CAD build for the part. Positions are in the model's coordinates, mm. A direction names the side the tool comes from. Round coordinates to 2 decimals unless told otherwise and drop trailing zeros. Order: outer loops, then holes, each group sorted by start corner. A loop starts at its lowest first (then second) coordinate and runs counter-clockwise, first axis right, second up. Notation, with made-up numbers: (44, -30.75) - (59, -30.75) arc R24 cw to (59, 4.25) - close; hole circle Ø2 at (32.25, 16.25). An arc over 180 degrees is marked (long way). Write item = value, one per line.
from build123d import *

# Parameters (mm, degrees)
SKETCH1_W           = 155
SKETCH1_H           = 32
BOSS_EXTRUDE1_DEPTH = 2
SKETCH2_W           = 155
SKETCH2_H           = 2
SKETCH2_W_2         = 130
BOSS_EXTRUDE2_DEPTH = 6.25
CUT_EXTRUDE1_DEPTH  = 6.25
SKETCH4_R           = 1.5
CUT_EXTRUDE2_DEPTH  = 6.25
SKETCH5_R           = 2.875
CUT_EXTRUDE3_DEPTH  = 6.25
SKETCH6_R           = 1.5
CUT_EXTRUDE4_DEPTH  = 6
CHAMFER1_SIZE       = 1.5


with BuildPart() as part:
    # Sketch1 → Boss-Extrude1 (new body)
    with BuildSketch(Plane.XY):
        with Locations((77.5, -16)):
            Rectangle(SKETCH1_W, SKETCH1_H)
    extrude(amount=BOSS_EXTRUDE1_DEPTH)

    # Sketch2 → Boss-Extrude2 (add)
    with BuildSketch(Plane.XY.offset(2)):
        with Locations((77.5, -1)):
            Rectangle(SKETCH2_W, SKETCH2_H)
        with Locations((90, -23)):
            Rectangle(SKETCH2_W_2, SKETCH2_H)
    extrude(amount=BOSS_EXTRUDE2_DEPTH)

    # Sketch3 → Cut-Extrude1 (cut)
    with BuildSketch(Plane.XY.offset(2)):
        Polygon((155, -32), (23, -32), (23, -24), (23, -20.25), (25, -20.25), (25, -24), (155, -24), align=None)
    extrude(amount=-CUT_EXTRUDE1_DEPTH, mode=Mode.SUBTRACT)

    # Sketch4 → Cut-Extrude2 (cut)
    with BuildSketch(Plane.XY.offset(2)):
        with Locations((4.75, -27.5)):
            Circle(SKETCH4_R)
        with Locations((4.75, -17.5)):
            Circle(SKETCH4_R)
        with Locations((4.75, -7.5)):
            Circle(SKETCH4_R)
    extrude(amount=-CUT_EXTRUDE2_DEPTH, mode=Mode.SUBTRACT)

    # Sketch5 → Cut-Extrude3 (cut)
    with BuildSketch(Plane.XY.offset(2)):
        with Locations((130.075, -12)):
            Circle(SKETCH5_R)
        with Locations((100.025, -12)):
            Circle(SKETCH5_R)
        with Locations((80.025, -12)):
            Circle(SKETCH5_R)
        with Locations((49.925, -12)):
            Circle(SKETCH5_R)
    extrude(amount=-CUT_EXTRUDE3_DEPTH, mode=Mode.SUBTRACT)

    # Sketch6 → Cut-Extrude4 (cut)
    with BuildSketch(Plane.XY.offset(2)):
        with Locations((14.75, -26)):
            Circle(SKETCH6_R)
        with Locations((14.75, -6)):
            Circle(SKETCH6_R)
        with Locations((34.75, -6)):
            Circle(SKETCH6_R)
    extrude(amount=-CUT_EXTRUDE4_DEPTH, mode=Mode.SUBTRACT)

    # Chamfer1
    chamfer1_edges = [part.edges().sort_by_distance(p)[0] for p in [
        (33.25, -6, 2),
    ]]
    chamfer(chamfer1_edges, length=CHAMFER1_SIZE)


solid = part.part
(1) Tool access for faces 1 (the flat face through (89, -22, 5)), 2 (the flat face through (89, -24, 4)), 3 (the flat face through (25, -23, 3)): list every direction of +Z, -Z, +X, -X, +Y, -Y with a clear straight run to the whole face (end or side of a thin tool).
Solved:
face_1 = +Z, +X, -X
face_2 = +Z, -Z, +X, -Y
face_3 = +Z, -Z, -Y
(2) Pull direction X, two halves, no side cores. Call faces 4 (the flat face through (0, -14, 1)), 5 (the flat face through (155, -12, 1)), 6 (the flat face through (76, -12, 0)), 7 (the cylindrical face through (127.2, -11.9, 1)): released by +X, released by -X, zero draft, split by the parting line, or undercut.
Solved:
face_4 = released by -X
face_5 = released by +X
face_6 = zero draft
face_7 = undercut
(3) Probe line 1 along Y through (x, z) = (14.75, 1.5); line 2 along Y through (x, z) = (75, 3.5); line 3 along Z through (x, y) = (132.5, -9). List the from-to ranges inside material, lowest first.
Solved:
line_1 = -32 to -27.5, -24.5 to -7.5, -4.5 to 0
line_2 = -24 to -22, -2 to 0
line_3 = 0 to 2
(4) Band-saw the part on D-D on x = 34.75. List the corners of the cut face in (y, z), plus the area to 4 significant figures.
Solved:
outline = (-24, 0) - (-7.5, 0) - (-7.5, 0.5) - (-9, 2) - (-22, 2) - (-22, 8.25) - (-24, 8.25) - close; (-4.5, 0) - (0, 0) - (0, 8.25) - (-2, 8.25) - (-2, 2) - (-3, 2) - (-4.5, 0.5) - close
area = 64.75 mm²
(5) Band-saw the part on C-C on z = 5. List the corners of the cut face in (x, y).
Solved:
outline = (0, -2) - (155, -2) - (155, 0) - (0, 0) - close; (25, -24) - (155, -24) - (155, -22) - (25, -22) - close
(6) Band-saw the part on B-B on y = -17.5. List the corners of the cut face in (x, z).
Solved:
outline = (0, 0) - (3.25, 0) - (3.25, 2) - (0, 2) - close; (6.25, 0) - (155, 0) - (155, 2) - (6.25, 2) - close
(7) Band-saw the part on A-A on x = 4.75. List the corners of the cut face in (y, z), plus the area to 3 significant figures.
Solved:
outline = (-32, 0) - (-29, 0) - (-29, 2) - (-32, 2) - close; (-26, 0) - (-19, 0) - (-19, 2) - (-26, 2) - close; (-16, 0) - (-9, 0) - (-9, 2) - (-16, 2) - close; (-6, 0) - (0, 0) - (0, 8.25) - (-2, 8.25) - (-2, 2) - (-6, 2) - close
area = 58.5 mm²
(8) Drop flat-ended pins along their axis: pin 1 (3.5 mm diameter, centred on x = 130.075, y = -12, fed in from +Z); pin 2 (0.6 mm diameter, centred on y = -27.5, z = 1, fed in from +X); pin 3 (2.5 mm diameter, centred on x = 119, z = 4, fed in from -Y); pin 4 (1.6 mm diameter, centred on x = 24, z = 1, fed in from -Y). Give the stop position or say it passes through.
Solved:
pin_1 = through
pin_2 = 23
pin_3 = -24
pin_4 = -20.25
